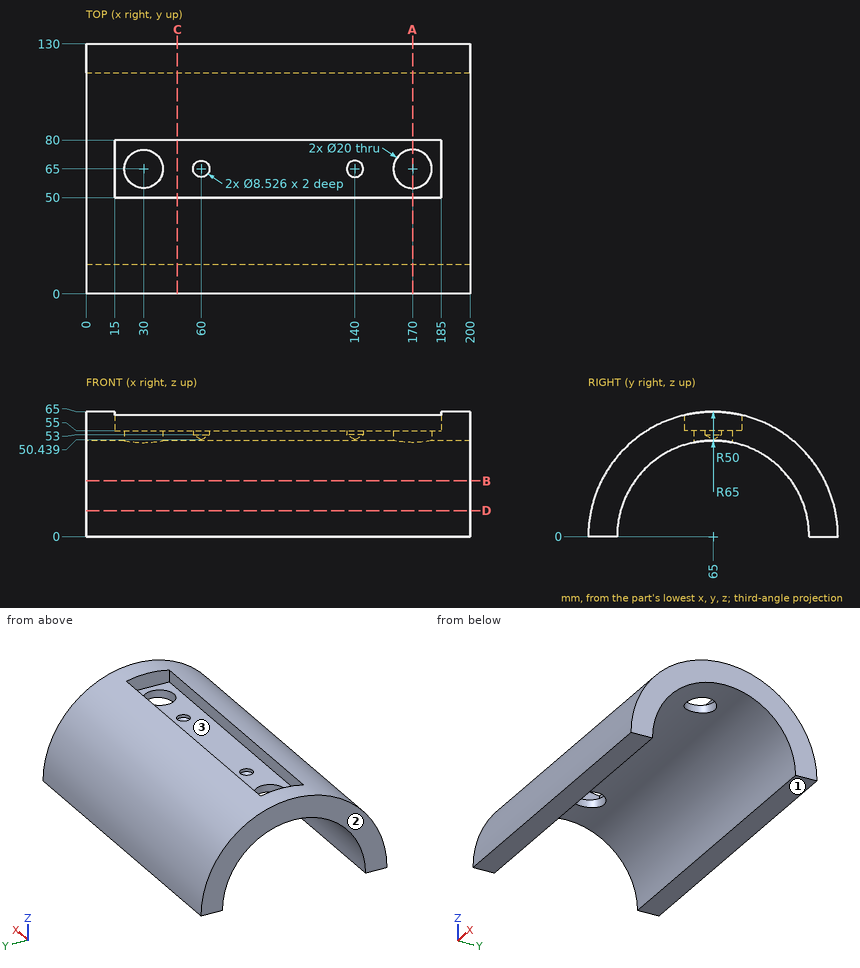
The drawing under review shows one solid part. Ordinate dimensions are in mm from its lowest x, y, z. Coordinates: 2 decimals unless noted, no trailing zeros. Order: outer loops, then holes, each group sorted by start corner. A loop starts at its lowest first (then second) coordinate and runs counter-clockwise, first axis right, second up. Notation, with made-up numbers: M 85,-37 L 139,-37 A6 ccw 139,-33 Z; hole C 51.25,29 d8. An arc over 180 degrees is marked long. Use a Markdown table: item, result.
(1) Add section C-C (x = 47.5). Give the boundary of the cut face in (y, z) (1 decimal), then the cut area to 3 significant figures.
Worked answers:
| item | result |
|---|---|
| outline | M 0,0 L 15,0 A50 cw 115,0 L 130,0 A65 ccw 80,63.2 L 80,55 L 50,55 L 50,63.2 A65 ccw Z |
| area | 2,430 mm2 |
(2) Draft analysis for pull direction X (two halves, no side actions). For the marked faces 1, 2 and 3, state which applies: released by +X, released by -X, zero draft, split by the parting line, or undercut.
Worked answers:
| item | result |
|---|---|
| face 1 | zero draft |
| face 2 | released by -X |
| face 3 | undercut |
(3) For P1, Ø2.5, axis at x = 113, z = 60, coming from the +Y side; P2, Ø2.5, axis at x = 65, z = 58, coming from the -Y side (1 decimal); P3, Ø2, axis at x = 135.5, z = 13, coming from the -Y side; P4, Ø1, axis at y = 106, z = 51.5, coming from the -X side, all flat-tipped, find the tip position at first contact; note any pin that passes through.
Worked answers:
| item | result |
|---|---|
| P1 | stops at y = 92.81 |
| P2 | stops at y = 33.3 |
| P3 | stops at y = 1.12 |
| P4 | passes through |
(4) Add section D-D (z = 13.5). Give the boundary of the cut face in (x, y).
Worked answers:
| item | result |
|---|---|
| outline | M 0,1.42 L 200,1.42 L 200,16.86 L 0,16.86 Z; M 0,113.14 L 200,113.14 L 200,128.58 L 0,128.58 Z |
(5) Add section A-A (x = 170). Give the boundary of the cut face in (y, z) (1 decimal), then the cut area to 3 significant figures.
Worked answers:
| item | result |
|---|---|
| outline | M 0,0 L 15,0 A50 cw 55,49 L 55,55 L 50,55 L 50,63.2 A65 ccw Z; M 75,49 A50 cw 115,0 L 130,0 A65 ccw 80,63.2 L 80,55 L 75,55 Z |
| area | 2,320 mm2 |
(6) Wall thickness on probe 1 along X at (y, z) = (65, 53.5); probe 2 along X at (y, z) = (65, 52.25) (1 decimal); probe 3 along X at (y, z) = (56.5, 54.5) (1 decimal): over which ranges is each line inside the solid? List them lowest first.
Worked answers:
| item | result |
|---|---|
| probe 1 | x = 0 to 20, 40 to 55.74, 64.26 to 135.74, 144.26 to 160, 180 to 200 |
| probe 2 | x = 0 to 20, 40 to 57, 63 to 137, 143 to 160, 180 to 200 |
| probe 3 | x = 0 to 24.7, 35.3 to 164.7, 175.3 to 200 |
(7) Add section B-B (z = 29). Give the boundary of the cut face in (x, y), then the cut area to 3 significant figures.
Worked answers:
| item | result |
|---|---|
| outline | M 0,6.83 L 200,6.83 L 200,24.27 L 0,24.27 Z; M 0,105.73 L 200,105.73 L 200,123.17 L 0,123.17 Z |
| area | 6,980 mm2 |
